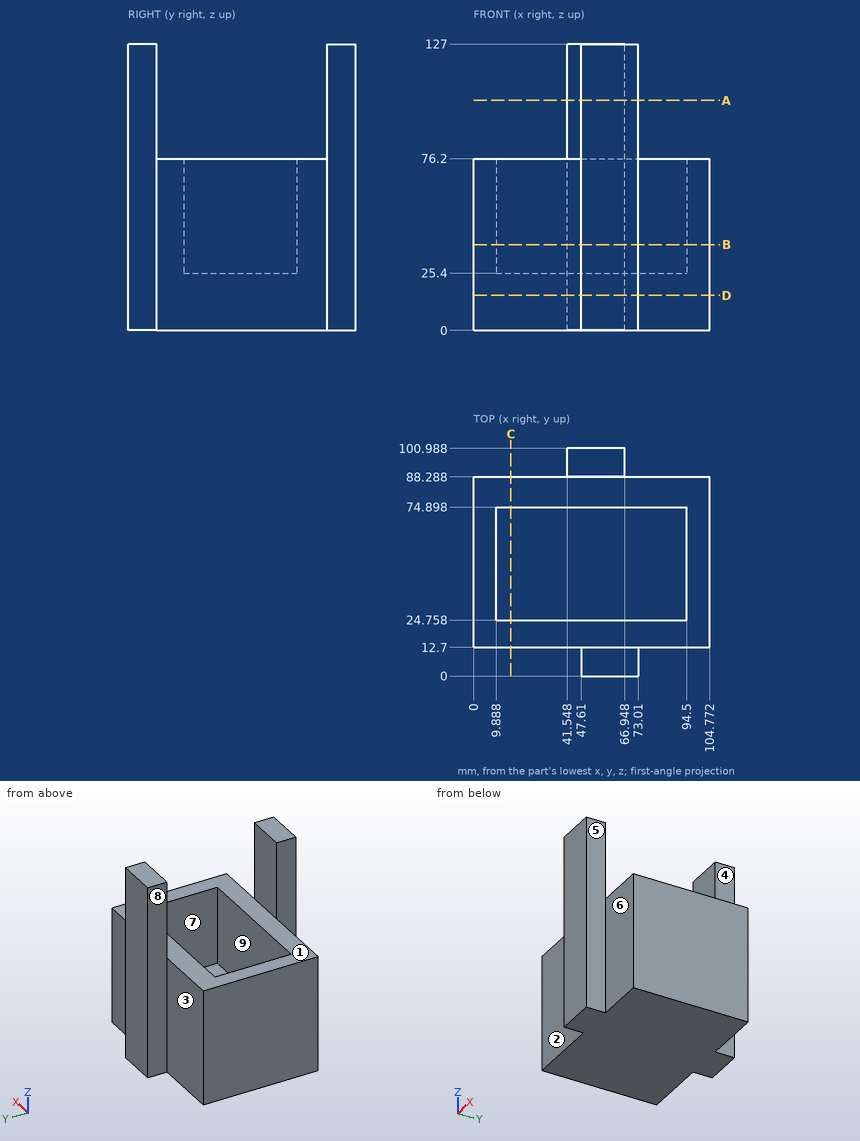
Study the drawing (mm; zero at the part's minimum x, y, z) and answer. A direction names the side the tool comes from. Give positions to 0.01 mm unless a question says otherwise; leave off trailing zeros. Order: outer loops, then holes, each group sorted by start corner. A loop starts at its lowest first (then second) coordinate and runs counter-clockwise, first axis right, second up. Notation, with made-up numbers: (-7.5, -38.5) -> (24.5, -38.5) arc R7 cw to (24.5, -30.5) -> close; hole circle Ø6 at (72.25, 17.25). An arc over 180 degrees is marked (long way). Write item = value, one per line.
1. A cutting plane is placed at A-A, the plane z = 102. Write down the section's boundary in (x, y), and give its area (3 significant figures).
Numbers:
outline = (41.55, 88.29) -> (66.95, 88.29) -> (66.95, 100.99) -> (41.55, 100.99) -> close; (47.61, 0) -> (73.01, 0) -> (73.01, 12.7) -> (47.61, 12.7) -> close
area = 645 mm²
2. A cutting plane is placed at C-C, the plane x = 16.5. Write down the section's boundary in (y, z), and give its area (3 significant figures).
Numbers:
outline = (12.7, 0) -> (88.29, 0) -> (88.29, 76.2) -> (74.9, 76.2) -> (74.9, 25.4) -> (24.76, 25.4) -> (24.76, 76.2) -> (12.7, 76.2) -> close
area = 3,210 mm²
3. For the marked faces 1, 2, 3, 4 and 5, determine the directions among +Z, -Z, +X, -X, +Y, -Y from which every point of the face is accessible in a straight line to the end or side of a thin tool.
Numbers:
face_1 = +Z, +X, -X
face_2 = +Z, -Z, -X, -Y
face_3 = +Z, -Z, -X, +Y
face_4 = +Z, -Z, +X, +Y
face_5 = +Z, -Z, +X, -Y
4. A cutting plane is placed at B-B, the plane z = 38. Write down the section's boundary in (x, y), and give its area (3 significant figures).
Numbers:
outline = (0, 12.7) -> (47.61, 12.7) -> (47.61, 0) -> (73.01, 0) -> (73.01, 12.7) -> (104.77, 12.7) -> (104.77, 88.29) -> (66.95, 88.29) -> (66.95, 100.99) -> (41.55, 100.99) -> (41.55, 88.29) -> (0, 88.29) -> close; hole (9.89, 24.76) -> (94.5, 24.76) -> (94.5, 74.9) -> (9.89, 74.9) -> close
area = 4,320 mm²
5. Straight lines are drawn through the part: line 1 along Y through (x, z) = (54, 56); line 2 along X through (y, z) = (45.5, 42); line 3 along Y through (x, z) = (36, 62). For each, find the intervals that lie inside material, in ascending order.
Numbers:
line_1 = 0 to 24.76, 74.9 to 100.99
line_2 = 0 to 9.89, 94.5 to 104.77
line_3 = 12.7 to 24.76, 74.9 to 88.29
6. A cutting plane is placed at D-D, the plane z = 15.5. Write down the section's boundary in (x, y).
Numbers:
outline = (0, 12.7) -> (47.61, 12.7) -> (47.61, 0) -> (73.01, 0) -> (73.01, 12.7) -> (104.77, 12.7) -> (104.77, 88.29) -> (66.95, 88.29) -> (66.95, 100.99) -> (41.55, 100.99) -> (41.55, 88.29) -> (0, 88.29) -> close
7. Given pin 1 (22.5 mm diameter, centred on x = 43.5, y = 53, fed in from +Z); pin 2 (4 mm diameter, centred on x = 67.5, z = 38, fed in from +Y); pin 3 (9.5 mm diameter, centred on x = 85, z = 55.5, fed in from -Y); pin 4 (14 mm diameter, centred on y = 6.5, z = 89, fed in from +X), each flat-ended and moving along its own axis, determine where each tip first touches the part or whether it passes through.
Numbers:
pin_1 = 25.4
pin_2 = 100.99
pin_3 = 12.7
pin_4 = 73.01
8. The mould has two halves that part along X. Classify the marked faces 6, 7, 8 and 9: +X half, -X half, draft (parallel to the pull), parting line (faces both ways), or undercut.
Numbers:
face_6 = draft
face_7 = undercut
face_8 = -X half
face_9 = undercut
